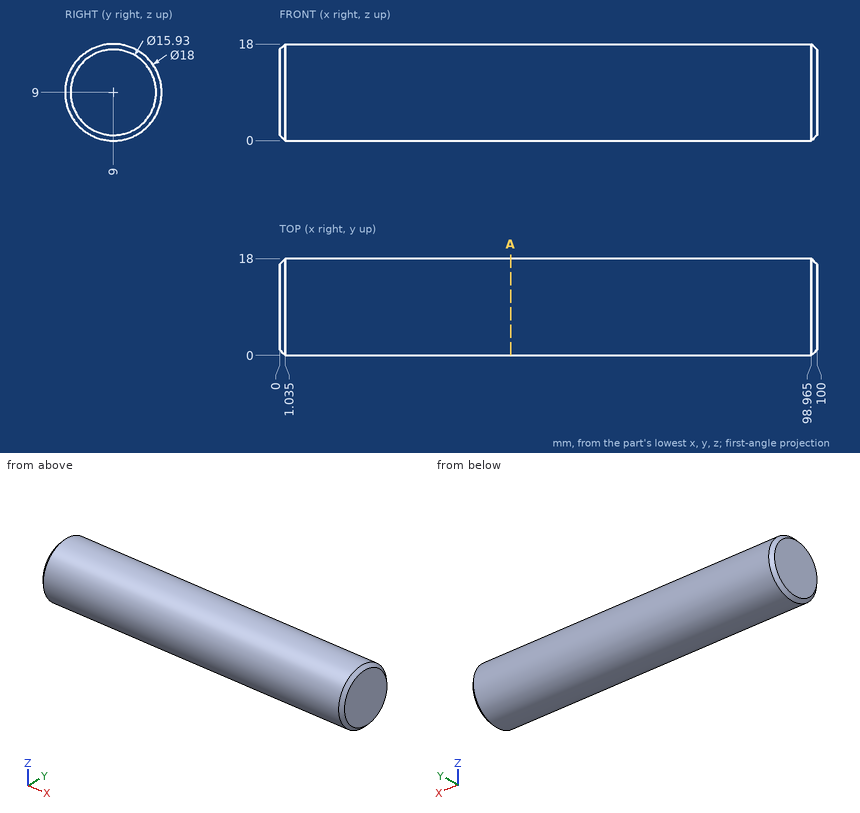
Verification items for this drawing (mm, ordinates from the low corner). Coordinates: 2 decimals unless noted, no trailing zeros. Write each loop counter-clockwise with the first axis right and the second up, starting at its lowest first coordinate (ties: lowest second). Pieces come first, ordered by that corner, then holes. Notation, with made-up numbers: (54, 59) - (95, 59) arc R18 cw to (95, 84) - close; hole circle Ø1 at (17, 45.5). An arc over 180 degrees is marked (long way). One line per question, with ' | ' between items.
Item 1: Sectioned sample at A-A on x = 43. Record the boundary of the cut face in (y, z).
Determined:
outline: circle Ø18 at (9, 9)
Item 2: Thickness scan on line 1 (Z direction, x = 54, y = 9.25); line 2 (Z direction, x = 49.5, y = 12); line 3 (Y direction, x = 53.5, z = 13). Record the ranges inside material, lowest first. Write a range as [from, to].
Determined:
line 1: z = [0, 18] | line 2: z = [0.51, 17.49] | line 3: y = [0.94, 17.06]
Item 3: Gauge pin test, flat ends, axial feed: P1, Ø2, axis at x = 48.5, y = 15, coming from the -Z side; P2, Ø6, axis at x = 84.5, y = 2, coming from the +Z side; P3, Ø4, axis at x = 77.5, z = 15, coming from the +Y side. Record the tip position at first contact, or that the pin passes through.
Determined:
P1: stops at z = 1.52 | P2: stops at z = 17.06 | P3: stops at y = 17.06
